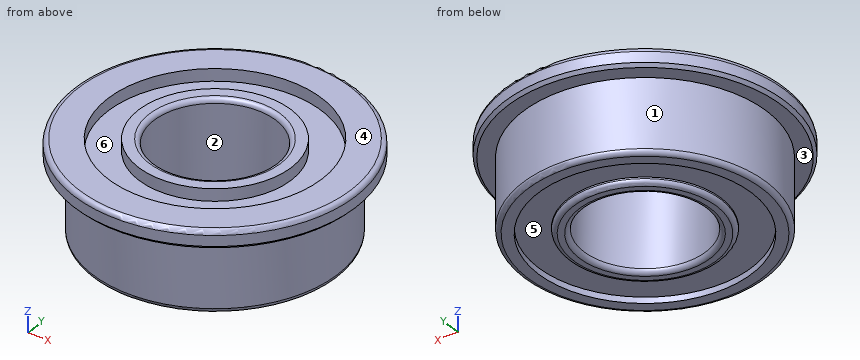
```python
from build123d import *

# Parameters (mm, degrees)
SKETCH1_R           = 4
SKETCH1_R_2         = 2
BOSS_EXTRUDE1_DEPTH = 3
BOSS_EXTRUDE2_START = -0.6
SKETCH2_R           = 4.6
SKETCH2_R_2         = 4
BOSS_EXTRUDE2_DEPTH = 0.6
SKETCH3_R           = 3.5
SKETCH3_R_2         = 2.5
CUT_EXTRUDE1_DEPTH  = 0.2
CUT_EXTRUDE2_START  = -2.6
SKETCH3_2_R         = 3.5
SKETCH3_2_R_2       = 2.5
CUT_EXTRUDE2_DEPTH  = 0.4
FILLET1_R           = 0.15
CHAMFER1_SIZE       = 0.1


with BuildPart() as part:
    # Sketch1 → Boss-Extrude1 (new body)
    with BuildSketch(Plane.XY):
        Circle(SKETCH1_R)
        Circle(SKETCH1_R_2, mode=Mode.SUBTRACT)
    extrude(amount=BOSS_EXTRUDE1_DEPTH)

    # Sketch2 → Boss-Extrude2 (add)
    with BuildSketch(Plane.XY.offset(3).offset(BOSS_EXTRUDE2_START)):
        Circle(SKETCH2_R)
        Circle(SKETCH2_R_2, mode=Mode.SUBTRACT)
    extrude(amount=BOSS_EXTRUDE2_DEPTH)

    # Sketch3 → Cut-Extrude1 (cut)
    with BuildSketch(Plane(origin=(0, 0, 0), x_dir=(-1, 0, 0), z_dir=(0, 0, -1))):
        Circle(SKETCH3_R)
        Circle(SKETCH3_R_2, mode=Mode.SUBTRACT)
    extrude(amount=-CUT_EXTRUDE1_DEPTH, mode=Mode.SUBTRACT)

    # Sketch3<2> → Cut-Extrude2 (cut)
    with BuildSketch(Plane(origin=(0, 0, 0), x_dir=(-1, 0, 0), z_dir=(0, 0, -1)).offset(CUT_EXTRUDE2_START)):
        Circle(SKETCH3_2_R)
        Circle(SKETCH3_2_R_2, mode=Mode.SUBTRACT)
    extrude(amount=-CUT_EXTRUDE2_DEPTH, mode=Mode.SUBTRACT)

    # Fillet1
    fillet1_edges = [part.edges().sort_by_distance(p)[0] for p in [
        (-4.6, 0, 3),
        (2.5, 0, 0),
        (-4, 0, 0),
        (-2, 0, 0),
        (-2, 0, 3),
    ]]
    fillet(fillet1_edges, radius=FILLET1_R)

    # Chamfer1
    chamfer1_edges = [part.edges().sort_by_distance(p)[0] for p in [
        (-4.6, 0, 2.4),
    ]]
    chamfer(chamfer1_edges, length=CHAMFER1_SIZE)


solid = part.part
```
Check sheet for the modelled part. Datum: model origin and axes. Units: mm. Face numbers are marked on the shaded views. A direction names the side the tool comes from. Coordinates: 2 decimals unless noted, no trailing zeros. Order: outer loops, then holes, each group sorted by start corner. A loop starts at its lowest first (then second) coordinate and runs counter-clockwise, first axis right, second up. Notation, with made-up numbers: (25.25, -38) -> (29.25, -38) arc R8 cw to (29.25, -31) -> close; hole circle Ø8 at (-17, 60). An arc over 180 degrees is marked (long way). Write item = value, one per line. Start each with the question number.
1) Mould release check, pull along Y, two halves, no side actions. Record for the marked faces 1, 2 and 3: +Y half, -Y half, draft (parallel to the pull), parting line (faces both ways), or undercut.
2) Access from +Z, -Z, +X, -X, +Y, -Y to the whole of each face (thin tool, end or side, straight path). Record for the marked faces 4, 5 and 6.
3) Cross-section at A-A (z = 0.7). Enter the section's corners in (x, y).
4) Go/stop test with flat-tipped pins: P1, Ø3.5, axis at x = 0.5, y = 0, coming from the +Z side; P2, Ø2.5, axis at x = 0, y = 0, coming from the -Z side. Record where each tip stops, or that it passes through.
5) Material ranges on L1, parallel to Y at x = 0, z = 0.95; L2, parallel to Y at x = 0, z = 0.1; L3, parallel to Z at x = -3, y = -3, recorded low to high.
Ans:
q1.face_1 = parting line
q1.face_2 = undercut
q1.face_3 = draft
q2.face_4 = +Z, +X, -X, +Y, -Y
q2.face_5 = -Z
q2.face_6 = +Z
q3.outline = circle Ø8 at (0, 0); hole circle Ø4 at (0, 0)
q4.P1 = 3
q4.P2 = through
q5.L1 = -4 to -2, 2 to 4
q5.L2 = -3.99 to -3.5, -2.49 to -2.01, 2.01 to 2.49, 3.5 to 3.99
q5.L3 = 2.4 to 3
